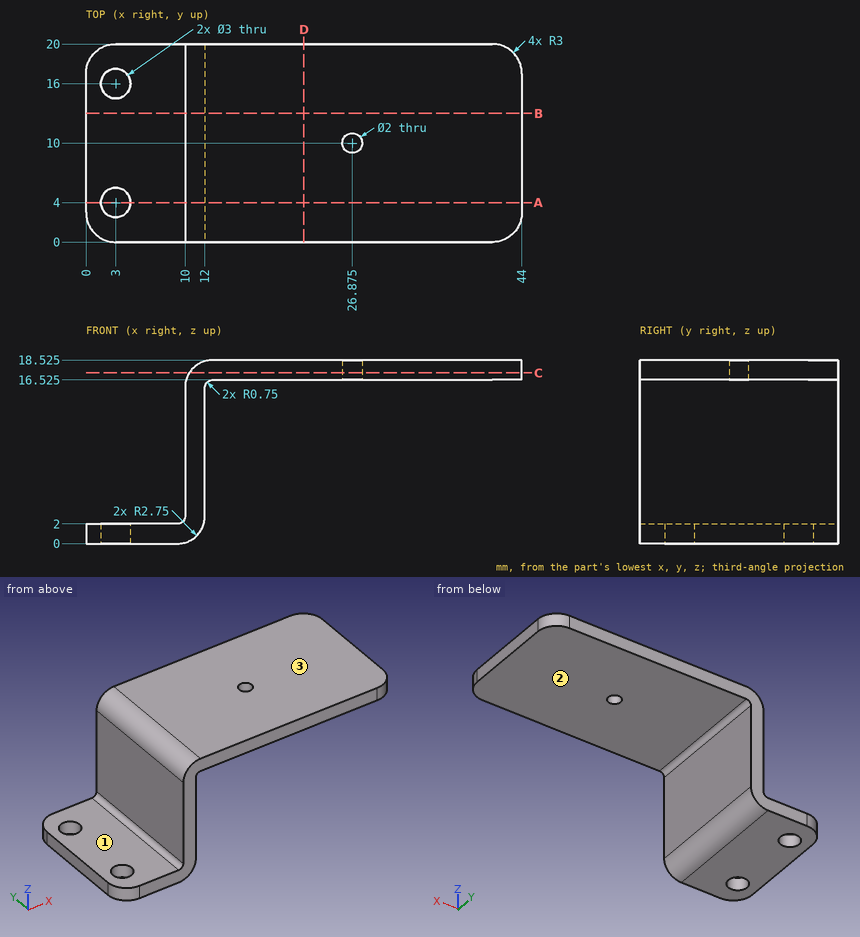
Source: three-view drawing plus pictorial views. Frame: mm from the lowest corner of the part. A direction names the side the tool comes from. Round coordinates to 2 decimals unless told otherwise and drop trailing zeros. Write each loop counter-clockwise with the first axis right and the second up, starting at its lowest first coordinate (ties: lowest second). Pieces come first, ordered by that corner, then holes. Notation, with made-up numbers: (75.5, -18) -> (124.5, -18) arc R10 cw to (124.5, -2) -> close; hole circle Ø1 at (83.5, 61). An arc over 180 degrees is marked (long way). Return JSON: item names as keys, results as strings.
Q1. First-contact query: pin 1 Ø6.5 at (y, z) = (11.5, 9) entering from +X; pin 2 Ø2.5 at (x, y) = (3, 4) entering from +Z; pin 3 Ø10.5 at (y, z) = (15, 11.5) entering from -X; pin 4 Ø3 at (x, y) = (5, 6) entering from +Z. Flat tips, straight axial feed; report the tip coordinate or a pass-through.
From the geometry:
{"pin 1": "x = 12", "pin 2": "through", "pin 3": "x = 10", "pin 4": "z = 2"}
Q2. Section B-B on y = 13. Return the cut outline in (x, z) (3 decimals).
From the geometry:
{"outline": "(0, 0) -> (9.25, 0) arc R2.75 ccw to (12, 2.75) -> (12, 15.775) arc R0.75 cw to (12.75, 16.525) -> (44, 16.525) -> (44, 18.525) -> (12.75, 18.525) arc R2.75 ccw to (10, 15.775) -> (10, 2.75) arc R0.75 cw to (9.25, 2) -> (0, 2) -> close"}
Q3. Set-up query: the marked faces 1, 2 and 3. Return all of +Z, -Z, +X, -X, +Y, -Y with unobstructed straight access to the full face (end or side cutting, diameter ignored); none if empty.
From the geometry:
{"face 1": "+Z, -X, +Y, -Y", "face 2": "-Z, +X, +Y, -Y", "face 3": "+Z, +X, -X, +Y, -Y"}
Q4. Section C-C on z = 17.25. Return the cut outline in (x, y) (3 decimals).
From the geometry:
{"outline": "(10.429, 0) -> (41, 0) arc R3 ccw to (44, 3) -> (44, 17) arc R3 ccw to (41, 20) -> (10.429, 20) -> close; hole circle Ø2 at (26.875, 10)"}
Q5. Section D-D on x = 22. Return the cut outline in (y, z) (3 decimals), and give its area (3 significant figures).
From the geometry:
{"outline": "(0, 16.525) -> (20, 16.525) -> (20, 18.525) -> (0, 18.525) -> close", "area": "40.0 mm2"}
Q6. Section A-A on y = 4. Return the cut outline in (x, z) (3 decimals), and give its area (3 significant figures).
From the geometry:
{"outline": "(0, 0) -> (1.5, 0) -> (1.5, 2) -> (0, 2) -> close; (4.5, 0) -> (9.25, 0) arc R2.75 ccw to (12, 2.75) -> (12, 15.775) arc R0.75 cw to (12.75, 16.525) -> (44, 16.525) -> (44, 18.525) -> (12.75, 18.525) arc R2.75 ccw to (10, 15.775) -> (10, 2.75) arc R0.75 cw to (9.25, 2) -> (4.5, 2) -> close", "area": "112 mm2"}
Q7. Ray query, line 1 (Y direction, x = 3, z = 0.65); line 2 (X direction, y = 3.75, z = 11.5); line 3 (Z direction, x = 3, y = 7). Return the intervals inside material, ascending.
From the geometry:
{"line 1": "0 to 2.5, 5.5 to 14.5, 17.5 to 20", "line 2": "10 to 12", "line 3": "0 to 2"}
